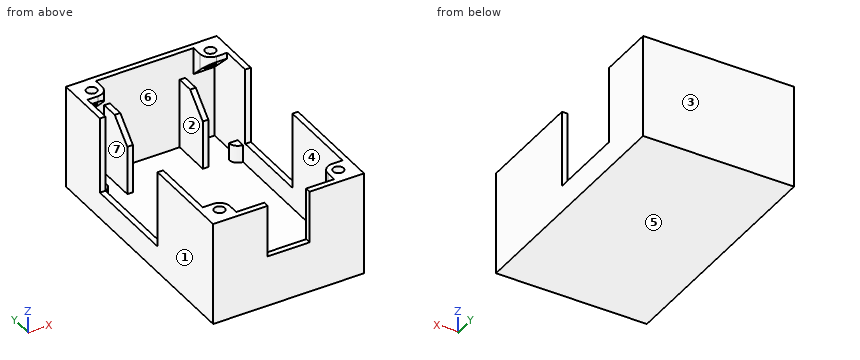
from build123d import *

# Parameters (mm, degrees)
SKETCH_W        = 43.2
SKETCH_H        = 70.2
PAD_DEPTH       = 1.6
SKETCH001_W     = 43.2
SKETCH001_H     = 70.2
SKETCH001_W_2   = 40
SKETCH001_H_2   = 67
PAD001_DEPTH    = 28
PAD002_DEPTH    = 5
SKETCH003_W     = 1.6
SKETCH003_H     = 27.5
SKETCH003_H_2   = 22.5
POCKET_DEPTH    = 22
SKETCH004_W     = 1.6
SKETCH004_H     = 11
PAD003_DEPTH    = 20
SKETCH005_W     = 12
SKETCH005_H     = 1.6
POCKET001_DEPTH = 15
SKETCH006_W     = 6
SKETCH006_H     = 6
PAD004_DEPTH    = 7.6
CHAMFER_SIZE    = 5.9
SKETCH007_R     = 1.5
POCKET002_DEPTH = 10
FILLET_R        = 3
CHAMFER001_SIZE = 6


with BuildPart() as part:
    # Sketch → Pad (new body)
    with BuildSketch(Plane.XY):
        with Locations((21.6, 35.1)):
            Rectangle(SKETCH_W, SKETCH_H)
    extrude(amount=PAD_DEPTH)

    # Sketch001 (on Face6 of Pad) → Pad001 (join)
    with BuildSketch(Plane.XY.offset(1.6)):
        with Locations((21.6, 35.1)):
            Rectangle(SKETCH001_W, SKETCH001_H)
        with Locations((21.6, 35.1)):
            Rectangle(SKETCH001_W_2, SKETCH001_H_2, mode=Mode.SUBTRACT)
    extrude(amount=PAD001_DEPTH)

    # Sketch002 (on Face15 of Pad001) → Pad002 (join)
    with BuildSketch(Plane.XY.offset(1.6)):
        with BuildLine():
            ThreePointArc((4.1, 1.6), (3.367767, 3.367767), (1.6, 4.1))
            Line((1.6, 4.1), (1.6, 1.6))
            Line((4.1, 1.6), (1.6, 1.6))
        make_face()
        with BuildLine():
            ThreePointArc((41.6, 4.1), (39.832233, 3.367767), (39.1, 1.6))
            Line((41.6, 1.6), (39.1, 1.6))
            Line((41.6, 4.1), (41.6, 1.6))
        make_face()
        with BuildLine():
            ThreePointArc((1.6, 55.1), (3.367767, 55.832233), (4.1, 57.6))
            Line((4.1, 57.6), (1.6, 57.6))
            Line((1.6, 55.1), (1.6, 57.6))
        make_face()
        with BuildLine():
            ThreePointArc((39.1, 57.6), (39.832233, 55.832233), (41.6, 55.1))
            Line((41.6, 55.1), (41.6, 57.6))
            Line((39.1, 57.6), (41.6, 57.6))
        make_face()
    extrude(amount=PAD002_DEPTH)

    # Sketch003 (on Face9 of Pad002) → Pocket (cut)
    with BuildSketch(Plane.XY.offset(29.6)):
        with Locations((0.8, 40.25)):
            Rectangle(SKETCH003_W, SKETCH003_H)
        with Locations((42.4, 42.75)):
            Rectangle(SKETCH003_W, SKETCH003_H_2)
    extrude(amount=-POCKET_DEPTH, mode=Mode.SUBTRACT)

    # Sketch004 (on Face22 of Pocket) → Pad003 (join)
    with BuildSketch(Plane.XY.offset(1.6)):
        with Locations((10.8, 63.1)):
            Rectangle(SKETCH004_W, SKETCH004_H)
        with Locations((32.4, 63.1)):
            Rectangle(SKETCH004_W, SKETCH004_H)
    extrude(amount=PAD003_DEPTH)

    # Sketch005 (on Face9 of Pad003) → Pocket001 (cut)
    with BuildSketch(Plane.XY.offset(29.6)):
        with Locations((21.6, 0.8)):
            Rectangle(SKETCH005_W, SKETCH005_H)
    extrude(amount=-POCKET001_DEPTH, mode=Mode.SUBTRACT)

    # Sketch006 (on Face13 of Pocket001) → Pad004 (join)
    with BuildSketch(Plane.XY.offset(29.6)):
        with Locations((4.6, 4.6)):
            Rectangle(SKETCH006_W, SKETCH006_H)
        with Locations((38.6, 4.6)):
            Rectangle(SKETCH006_W, SKETCH006_H)
        with Locations((4.6, 65.6)):
            Rectangle(SKETCH006_W, SKETCH006_H)
        with Locations((38.6, 65.6)):
            Rectangle(SKETCH006_W, SKETCH006_H)
    extrude(amount=-PAD004_DEPTH)

    # Chamfer
    chamfer_edges = [part.edges().sort_by_distance(p)[0] for p in [
        (38.6, 62.6, 22),
        (4.6, 62.6, 22),
        (38.6, 7.6, 22),
        (4.6, 7.6, 22),
    ]]
    chamfer(chamfer_edges, length=CHAMFER_SIZE)

    # Sketch007 → Pocket002 (cut)
    with BuildSketch(Plane.XY.offset(29.6)):
        with Locations((4.6, 4.6)):
            Circle(SKETCH007_R)
        with Locations((38.6, 4.6)):
            Circle(SKETCH007_R)
        with Locations((4.6, 65.6)):
            Circle(SKETCH007_R)
        with Locations((38.6, 65.6)):
            Circle(SKETCH007_R)
    extrude(amount=-POCKET002_DEPTH, mode=Mode.SUBTRACT)

    # Fillet
    fillet_edges = [part.edges().sort_by_distance(p)[0] for p in [
        (7.6, 62.6, 28.75),
        (35.6, 62.6, 28.75),
        (7.6, 7.6, 28.75),
        (35.6, 7.6, 28.75),
    ]]
    fillet(fillet_edges, radius=FILLET_R)

    # Chamfer001
    chamfer001_edges = [part.edges().sort_by_distance(p)[0] for p in [
        (10.8, 57.6, 21.6),
        (32.4, 57.6, 21.6),
    ]]
    chamfer(chamfer001_edges, length=CHAMFER001_SIZE)


solid = part.part
CAD build for the part. Positions are in the model's coordinates, mm. Face numbers are marked on the shaded views. A direction names the side the tool comes from. Round coordinates to 2 decimals unless told otherwise and drop trailing zeros. Loops run counter-clockwise (first coordinate to the right, second up) from the corner with the lowest first, then second, coordinate; pieces in that order, holes last. Notation, with made-up numbers: M 83,-15.75 L 91,-15.75 A21 cw 91,10.25 Z; hole C -2.5,85 d11. An arc over 180 degrees is marked long. One line per question, with ' | ' between items. Start each with the question number.
Item 1: Cut at D-D, the plane x = 14.5. Write the cut outline in (y, z).
Item 2: Cut at B-B, the plane y = 29.5. Write the cut outline in (x, z).
Item 3: Two-plate mould, pull along Y, no slides. Class the marked faces 1, 2, 3 and 4: pulls with the +Y half, pulls with the -Y half, needs draft (parallel to the pull), parting line crosses it, or undercut.
Item 4: Pin check, flat tips, straight feed: pin 1 Ø0.8 at (x, y) = (3.5, 56) entering from +Z; pin 2 Ø0.5 at (x, y) = (32.5, 66) entering from +Z; pin 3 Ø0.5 at (x, y) = (23.5, 0.5) entering from +Z; pin 4 Ø4 at (y, z) = (13, 14.5) entering from -X. Stop position of each tip, or through.
Item 5: Which spindle directions (+Z, -Z, +X, -X, +Y, -Y) get a long thin tool onto all of the face, cutting with end or side? Do the marked faces 5, 6 and 7. Say none if no direction does.
Item 6: Cut at A-A, the plane z = 18.25. Write the cut outline in (x, y), plus the area to 3 significant figures.
Item 7: Cut at C-C, the plane z = 12.25. Write the cut outline in (x, y).
Item 8: Wall check: line 1 (X direction, y = 66, z = 4); line 2 (X direction, y = 4.6, z = 26); line 3 (Y direction, x = 4.6, z = 28.25). Give the ranges that are in metal, low to high.
Responses:
1) outline: M 0,0 L 70.2,0 L 70.2,29.6 L 68.6,29.6 L 68.6,1.6 L 1.6,1.6 L 1.6,29.6 L 0,29.6 Z
2) outline: M 0,0 L 43.2,0 L 43.2,29.6 L 41.6,29.6 L 41.6,1.6 L 1.6,1.6 L 1.6,7.6 L 0,7.6 Z
3) face 1: needs draft | face 2: undercut | face 3: pulls with the +Y half | face 4: undercut
4) pin 1: stops at z = 6.6 | pin 2: stops at z = 21.6 | pin 3: stops at z = 14.6 | pin 4: stops at x = 0
5) face 5: -Z, +X, -X, +Y, -Y | face 6: none | face 7: +Z
6) outline: M 0,0 L 15.6,0 L 15.6,1.6 L 1.6,1.6 L 1.6,26.5 L 0,26.5 Z; M 0,54 L 1.6,54 L 1.6,68.6 L 10,68.6 L 10,60.25 L 11.6,60.25 L 11.6,68.6 L 31.6,68.6 L 31.6,60.25 L 33.2,60.25 L 33.2,68.6 L 41.6,68.6 L 41.6,54 L 43.2,54 L 43.2,70.2 L 0,70.2 Z; M 27.6,0 L 43.2,0 L 43.2,31.5 L 41.6,31.5 L 41.6,1.6 L 27.6,1.6 Z | area: 280 mm²
7) outline: M 0,0 L 43.2,0 L 43.2,31.5 L 41.6,31.5 L 41.6,1.6 L 1.6,1.6 L 1.6,26.5 L 0,26.5 Z; M 0,54 L 1.6,54 L 1.6,68.6 L 10,68.6 L 10,57.6 L 11.6,57.6 L 11.6,68.6 L 31.6,68.6 L 31.6,57.6 L 33.2,57.6 L 33.2,68.6 L 41.6,68.6 L 41.6,54 L 43.2,54 L 43.2,70.2 L 0,70.2 Z
8) line 1: x = 0 to 1.6, 10 to 11.6, 31.6 to 33.2, 41.6 to 43.2 | line 2: x = 0 to 3.1, 6.1 to 7.6, 35.6 to 37.1, 40.1 to 43.2 | line 3: y = 0 to 3.1, 6.1 to 7.6, 62.6 to 64.1, 67.1 to 70.2
